Geometry: final body of the model. Coordinates: model frame, mm. A direction names the side the tool comes from. Give positions to 0.01 mm unless a question says otherwise; leave off trailing zeros. Write each loop counter-clockwise with the first axis right and the second up, starting at its lowest first coordinate (ties: lowest second). Pieces come first, ordered by that corner, then holes.
Q1. Pin query (flat end, axial travel): pin 1 Ø3 at (y, z) = (28, 6.5) entering from -X; pin 2 Ø4 at (x, z) = (29.5, 18.5) entering from +Y; pin 3 Ø12 at (x, y) = (45, 42) entering from +Z; pin 4 Ø2 at (x, z) = (54.5, 15.5) entering from +Y. Return the tip coordinate at first contact, or that it passes through.
Q2. Section B-B (y = 12.5). Return the cut outline in (x, z), plus the area to 3 significant figures.
Q3. Line query: line 1 (Y direction, x = 35.5, z = 16.25); line 2 (X direction, y = 6.5, z = 16.5); line 3 (X direction, y = 16, z = 11). Output: solid intervals per line, ascending.
Q4. Reachability of faces 1 (the cylindrical face through (15.13, 2.63, 12.29)), 2 (the flat face through (34, 2.5, 11)), 3 (the cylindrical face through (30.8, 53.1, 13.5)), 4 (the cylindrical face through (52.58, 7.13, 12.79)) from +Z, -Z, +X, -X, +Y, -Y: full face, straight path, thin tool, end or side. Return the list, or none.
Q5. Section D-D (y = 54). Return the cut outline in (x, z).
Q6. Section A-A (x = 34). Return the cut outline in (y, z).
Q7. Section C-C (z = 18). Return the cut outline in (x, y), plus the area to 3 significant figures.
from build123d import *

# Parameters (mm, degrees)
BOX008_W                = 20
BOX008_H                = 43
BOX008_DEPTH            = 20
CYLINDER001_R           = 5.5
CYLINDER001_DEPTH       = 17.4
CYLINDER001_PITCH_ANGLE = 90
CYLINDER002_R           = 4
CYLINDER002_DEPTH       = 15.5
CYLINDER002_ROLL_ANGLE  = -90
CYLINDER_R              = 5.5
CYLINDER_DEPTH          = 17.5
CYLINDER_PITCH_ANGLE    = 90


with BuildPart() as e_valve_body:
    # Box008 → Box008 (new body)
    with BuildSketch(Plane(origin=(24, 0, 0), x_dir=(1, 0, 0), z_dir=(0, 0, 1))):
        with Locations((10, 21.5)):
            Rectangle(BOX008_W, BOX008_H)
    extrude(amount=BOX008_DEPTH)


with BuildPart() as o2out:
    # Cylinder001 → Cylinder001 (new body)
    with BuildSketch(Plane.XY):
        Circle(CYLINDER001_R)
    extrude(amount=CYLINDER001_DEPTH)


with BuildPart() as o2out_1:
    # Cylinder001 pitch: moved
    add(o2out.part.rotate(Axis((0, 0, 0), (0, 1, 0)), CYLINDER001_PITCH_ANGLE))


with BuildPart() as o2out_2:
    # Cylinder001 placement: moved
    add(o2out_1.part.moved(Location((44, 10, 10.5))))


with BuildPart() as o2sense:
    # Cylinder002 → Cylinder002 (new body)
    with BuildSketch(Plane.XY):
        Circle(CYLINDER002_R)
    extrude(amount=CYLINDER002_DEPTH)


with BuildPart() as o2sense_1:
    # Cylinder002 roll: moved
    add(o2sense.part.rotate(Axis((0, 0, 0), (1, 0, 0)), CYLINDER002_ROLL_ANGLE))


with BuildPart() as o2sense_2:
    # Cylinder002 placement: moved
    add(o2sense_1.part.moved(Location((34, 43, 10))))


with BuildPart() as e_valve:
    # Cylinder → Cylinder (new body)
    with BuildSketch(Plane.XY):
        Circle(CYLINDER_R)
    extrude(amount=CYLINDER_DEPTH)


with BuildPart() as e_valve_1:
    # Cylinder pitch: moved
    add(e_valve.part.rotate(Axis((0, 0, 0), (0, 1, 0)), CYLINDER_PITCH_ANGLE))


with BuildPart() as e_valve_2:
    # Cylinder placement: moved
    add(e_valve_1.part.moved(Location((6.5, 5.5, 10))))

    # Fusion: union e-valve body, O2out, O2sense
    add(e_valve_body.part)
    add(o2out_2.part)
    add(o2sense_2.part)


with BuildPart() as e_valve_3:
    # Fusion placement: moved
    add(e_valve_2.part.moved(Location((0, 2.5, 1.1))))


solid = e_valve_3.part
Computed:
1. pin 1: stops at x = 24
1. pin 2: stops at y = 45.5
1. pin 3: stops at z = 21.1
1. pin 4: stops at y = 17.17
2. outline: (6.5, 7.94) - (24, 7.94) - (24, 1.1) - (44, 1.1) - (44, 6.1) - (61.4, 6.1) - (61.4, 17.1) - (44, 17.1) - (44, 21.1) - (24, 21.1) - (24, 14.26) - (6.5, 14.26) - close
2. area: 702 mm2
3. line 1: y = 2.5 to 45.5
3. line 2: x = 24 to 44
3. line 3: x = 24 to 61.4
4. face 1: -X
4. face 2: +Z, -Z, +X, -X, -Y
4. face 3: +Y
4. face 4: +X
5. outline: circle Ø8 at (34, 11.1)
6. outline: (2.5, 1.1) - (45.5, 1.1) - (45.5, 7.1) - (61, 7.1) - (61, 15.1) - (45.5, 15.1) - (45.5, 21.1) - (2.5, 21.1) - close
7. outline: (24, 2.5) - (44, 2.5) - (44, 45.5) - (24, 45.5) - close
7. area: 860 mm2
